```python
from build123d import *

# Parameters (mm, degrees)
BOSS_EXTRUDE1_DEPTH = 16
CUT_EXTRUDE1_START  = 2
CUT_EXTRUDE1_DEPTH  = 14
SKETCH7_R           = 1.625
CUT_EXTRUDE2_DEPTH  = 55.539321396
CUT_EXTRUDE3_START  = -18
SKETCH8_W           = 10.868969255
SKETCH8_H           = 5.55
CUT_EXTRUDE3_DEPTH  = 2.5
SKETCH9_R           = 1.625
CUT_EXTRUDE4_DEPTH  = 8
SKETCH16_R          = 3.75
CUT_EXTRUDE9_DEPTH  = 3
SKETCH21_W          = 35
SKETCH21_H          = 21
CUT_EXTRUDE13_DEPTH = 2
FILLET2_R           = 0.5
FILLET3_R           = 3
FILLET4_R           = 1
CHAMFER3_SIZE       = 3.5
CHAMFER4_SIZE       = 4
SKETCH18_R          = 1.625
CUT_EXTRUDE11_DEPTH = 20
SKETCH19_R          = 4
CUT_EXTRUDE12_DEPTH = 5
CHAMFER9_SIZE       = 2
CHAMFER12_SIZE      = 1.5
CHAMFER11_SIZE      = 2


# Some blends are built 0.0001 mm under size
with BuildPart() as part:
    # Sketch4 → Boss-Extrude1 (new body)
    with BuildSketch(Plane.XY):
        Polygon((-3.5, -0.026126862), (-3.5, 6.973873138), (9, 6.973873138), (9, 12.473873138), (5.5, 12.473873138), (5.5, 27.973873138), (25.5, 27.973873138), (25.5, 15.473873138), (40.5, 15.473873138), (40.5, 9.473873138), (25.5, 9.473873138), (25.5, 6.973873138), (51.5, 6.973873138), (51.5, -0.026126862), align=None)
    extrude(amount=-BOSS_EXTRUDE1_DEPTH)

    # Sketch6 → Cut-Extrude1 (cut)
    with BuildSketch(Plane.XY.offset(CUT_EXTRUDE1_START)):
        with BuildLine():
            Line((12, 19.273873138), (5.5, 19.273873138))
            Line((5.5, 19.273873138), (5.5, 16.973873138))
            Line((5.5, 16.973873138), (20, 16.973873138))
            ThreePointArc((20, 16.973873138), (23.888996032, 18.58469458), (25.499999994, 22.473615007))
            Line((25.499999994, 22.473615007), (25.5, 27.973873138))
            Line((25.5, 27.973873138), (20, 27.973873138))
            ThreePointArc((20, 27.973873138), (17.189181506, 27.201377701), (15.167942816, 25.100891099))
            Line((15.167942816, 25.100891099), (12, 19.273873138))
        make_face()
        with BuildLine():
            Line((20, 18.673873138), (13.608794956, 18.673873138))
            Line((13.608794956, 18.673873138), (16.661487764, 24.28890373))
            ThreePointArc((16.661487764, 24.28890373), (23.26627588, 24.415893189), (20, 18.673873138))
        make_face(mode=Mode.SUBTRACT)
    extrude(amount=-CUT_EXTRUDE1_DEPTH, mode=Mode.SUBTRACT)

    # Sketch7 → Cut-Extrude2 (cut, through all)
    with BuildSketch(Plane(origin=(40.5, 0, 0), x_dir=(0, 0, -1), z_dir=(1, 0, 0))):
        with Locations((8, 12.473873138)):
            Circle(SKETCH7_R)
    extrude(amount=-CUT_EXTRUDE2_DEPTH, mode=Mode.SUBTRACT)

    # Sketch8 → Cut-Extrude3 (cut)
    with BuildSketch(Plane(origin=(40.5, 0, 0), x_dir=(0, 0, -1), z_dir=(1, 0, 0)).offset(CUT_EXTRUDE3_START)):
        with Locations((5.434484628, 12.473873138)):
            Rectangle(SKETCH8_W, SKETCH8_H)
    extrude(amount=-CUT_EXTRUDE3_DEPTH, mode=Mode.SUBTRACT)

    # Sketch9 → Cut-Extrude4 (cut)
    with BuildSketch(Plane.XZ.offset(0.026126862)):
        with Locations((3.5, -8)):
            Circle(SKETCH9_R)
        with Locations((44.5, -8)):
            Circle(SKETCH9_R)
    extrude(amount=-CUT_EXTRUDE4_DEPTH, mode=Mode.SUBTRACT)

    # Sketch16 → Cut-Extrude9 (cut)
    with BuildSketch(Plane(origin=(0, 6.973873138, 0), x_dir=(1, 0, 0), z_dir=(0, 1, 0))):
        with Locations(Location((3.5, 8, 0), (0, 0, 180))):
            Circle(SKETCH16_R)
        with Locations(Location((44.5, 8, 0), (0, 0, 180))):
            Circle(SKETCH16_R)
    extrude(amount=-CUT_EXTRUDE9_DEPTH, mode=Mode.SUBTRACT)

    # Sketch21 → Cut-Extrude13 (cut)
    with BuildSketch(Plane.XY):
        with Locations((23, 17.473873138)):
            Rectangle(SKETCH21_W, SKETCH21_H)
    extrude(amount=-CUT_EXTRUDE13_DEPTH, mode=Mode.SUBTRACT)

    # Fillet2
    fillet2_edges = [part.edges().sort_by_distance(p)[0] for p in [
        (20, 27.973873138, -7),
        (25.499999994, 22.473615007, -7),
    ]]
    fillet(fillet2_edges, radius=FILLET2_R)

    # Fillet3
    fillet3_edges = [part.edges().sort_by_distance(p)[0] for p in [
        (25.5, 27.973873138, -14),
    ]]
    fillet(fillet3_edges, radius=FILLET3_R)

    # Fillet4
    fillet4_edges = [part.edges().sort_by_distance(p)[0] for p in [
        (13.608794956, 18.673873138, -7),
    ]]
    fillet(fillet4_edges, radius=FILLET4_R)

    # Chamfer3
    # the kernel refuses this chamfer: 3.5 mm, written as the material it takes off along each edge
    with BuildSketch(Plane(origin=(5.5, 12.473873138, 7.000890458), x_dir=(-0.02749587661058662, 0.9996219169112968, 0), z_dir=(0, 0, -1))) as chamfer3_piece_1_section:
        Polygon((CHAMFER3_SIZE * 0.999621916911, CHAMFER3_SIZE * 0.0274958766106), (-CHAMFER3_SIZE * 0.0274958766106, CHAMFER3_SIZE * 0.999621916911), (0, 0), align=None)
    chamfer3_piece_1 = extrude(amount=22.376780916, mode=Mode.PRIVATE)
    chamfer3_piece_1 = split(chamfer3_piece_1, bisect_by=Plane(origin=(9, 13.630287679, -4.1875), z_dir=(-1, 0, 0)), keep=Keep.TOP, mode=Mode.PRIVATE)
    add(chamfer3_piece_1, mode=Mode.SUBTRACT)
    with BuildSketch(Plane(origin=(5.5, 12.473873138, -0.624109542), x_dir=(-0.02749587661058662, 0.9996219169112968, 0), z_dir=(0, 0, -1))) as chamfer3_piece_2_section:
        Polygon((CHAMFER3_SIZE * 0.999621916911, CHAMFER3_SIZE * 0.0274958766106), (-CHAMFER3_SIZE * 0.0274958766106, CHAMFER3_SIZE * 0.999621916911), (0, 0), align=None)
    chamfer3_piece_2 = extrude(amount=24.376780916, mode=Mode.PRIVATE)
    chamfer3_piece_2 = split(chamfer3_piece_2, bisect_by=Plane(origin=(9, 13.630287679, -12.8125), z_dir=(-1, 0, 0)), keep=Keep.TOP, mode=Mode.PRIVATE)
    add(chamfer3_piece_2, mode=Mode.SUBTRACT)

    # Chamfer4
    chamfer4_edges = [part.edges().sort_by_distance(p)[0] for p in [
        (5.5, 27.973873138, -9),
    ]]
    chamfer(chamfer4_edges, length=CHAMFER4_SIZE)

    # Sketch18 → Cut-Extrude11 (cut)
    with BuildSketch(Plane.XY):
        with Locations((20, 22.473873138)):
            Circle(SKETCH18_R)
    extrude(amount=-CUT_EXTRUDE11_DEPTH, mode=Mode.SUBTRACT)

    # Sketch19 → Cut-Extrude12 (cut)
    with BuildSketch(Plane(origin=(0, 16.973873138, 0), x_dir=(1, 0, 0), z_dir=(0, 1, 0))):
        with Locations((2.5, 8)):
            Circle(SKETCH19_R)
    extrude(amount=-CUT_EXTRUDE12_DEPTH, mode=Mode.SUBTRACT)

    # Chamfer9
    chamfer9_edges = [part.edges().sort_by_distance(p)[0] for p in [
        (17.25, 6.973873138, -2),
    ]]
    chamfer(chamfer9_edges, length=CHAMFER9_SIZE - 0.0001)  # a hair under: the kernel refuses the full size

    # Chamfer12
    # the kernel refuses this chamfer: 1.5 mm, written as the material it takes off along each edge
    with BuildSketch(Plane(origin=(23.857524482, 18.673873138, -2), x_dir=(0, 0.9996219169112968, 0.027495876610586334), z_dir=(-1, 0, 0))) as chamfer12_piece_1_section:
        Polygon((CHAMFER12_SIZE * 0.999621916911, CHAMFER12_SIZE * 0.0274958766106), (-CHAMFER12_SIZE * 0.0274958766106, CHAMFER12_SIZE * 0.999621916911), (0, 0), align=None)
    chamfer12_piece_1 = extrude(amount=12.424357944, mode=Mode.PRIVATE)
    chamfer12_piece_1 = split(chamfer12_piece_1, bisect_by=Plane(origin=(15.45343037, 22.066839589, -2.289421032), z_dir=(0.8785558517032834, -0.47763962925820797, 0)), keep=Keep.TOP, mode=Mode.PRIVATE)
    add(chamfer12_piece_1, mode=Mode.SUBTRACT)

    # Chamfer11
    chamfer11_edges = [part.edges().sort_by_distance(p)[0] for p in [
        (8.75, 19.273873138, -2),
    ]]
    chamfer(chamfer11_edges, length=CHAMFER11_SIZE)


solid = part.part
```
Here's how the part is built. I have some questions about the finished solid (model axes, mm). A direction names the side the tool comes from. Give positions to 0.01 mm unless a question says otherwise; leave off trailing zeros. Write each loop counter-clockwise with the first axis right and the second up, starting at its lowest first coordinate (ties: lowest second). Pieces come first, ordered by that corner, then holes. Notation, with made-up numbers: M 58,29.25 L 112,29.25 A10 cw 112,35.25 Z; hole C 88,26.5 d1. An arc over 180 degrees is marked long. Put each result on its own line as item: value. Start each with the question number.
Item 1: On a 3-axis mill with a long thin cutter (end or side, diameter ignored), from which of +Z, -Z, +X, -X, +Y, -Y can I reach the whole of each face in a straight line? I mean faces 4 (the flat face through (7.225, 14.248, -8.902)), 5 (the flat face through (21, 15.249, -6)), 6 (the flat face through (11, 25, -2)). Say none if no direction works.
Item 2: If we section it at D-D, the plane x = 4: Write out the boundary of the cut face in (y, z), then the cut area to 3 significant figures.
Item 3: If we section it at B-B, the plane y = 13.25: Write out the boundary of the cut face in (x, z), then the cut area to 3 significant figures.
Item 4: I need wall thicknesses on L1, parallel to Y at x = 36, z = -8; L2, parallel to X at y = 10, z = -10.5; L3, parallel to Y at x = 20, z = -12.25. Which ranges of each line are inside material? Lowest first, please. Write a range as from..to.
Item 5: Will these pins go through, and if not, where does the flat tip stop? pin 1 (3 mm diameter, centred on y = 11.5, z = -8, fed in from +X); pin 2 (3.5 mm diameter, centred on x = 44.5, z = -8, fed in from +Y); pin 3 (3.5 mm diameter, centred on x = 20, y = 22.47, fed in from +Z).
Item 6: Thinking about a two-plate mould opening in X: for faces 1 (the flat face through (51.5, 4, -8)), 2 (the flat face through (18, 18.674, -8)), 3 (the cylindrical face through (15.957, 26.203, -6.93)), which applies, +X half, -X half, draft (parallel to the pull), parting line (faces both ways), or undercut?
Item 7: If we section it at A-A, the plane x = 44.5: Write out the boundary of the cut face in (y, z) (3 decimals).
Item 8: If we section it at C-C, the plane z = -8: Count the separate pieces of the cut face and the enclosed holes in it, then the cut area to 3 significant figures.
Values:
1. face 4: +Z, -Z, -X
1. face 5: +Z
1. face 6: +Z, +X, -X, +Y
2. outline: M -0.03,-16 L 6.97,-16 L 6.97,-11.72 L 3.97,-11.72 L 3.97,-9.55 L -0.03,-9.55 Z; M -0.03,-6.45 L 3.97,-6.45 L 3.97,-4.28 L 6.97,-4.28 L 6.97,0 L -0.03,0 Z
2. area: 77.3 mm²
3. outline: M 8.22,-16 L 40.5,-16 L 40.5,-9.43 L 22.5,-9.43 L 22.5,-10.87 L 20,-10.87 L 20,-9.43 L 8.22,-9.43 Z; M 8.22,-6.57 L 20,-6.57 L 20,-2 L 8.22,-2 Z; M 22.5,-6.57 L 40.5,-6.57 L 40.5,-2 L 22.5,-2 Z
3. area: 345 mm²
4. L1: -0.03..6.97, 9.47..10.85, 14.1..15.47
4. L2: 9..20, 22.5..40.5
4. L3: -0.03..20.85, 24.1..27.97
5. pin 1: x = 40.5
5. pin 2: y = 3.97
5. pin 3: z = -2
6. face 1: +X half
6. face 2: draft
6. face 3: undercut
7. outline: M -0.026,-16 L 6.974,-16 L 6.974,-11.75 L 3.974,-11.75 L 3.974,-9.625 L -0.026,-9.625 Z; M -0.026,-6.375 L 3.974,-6.375 L 3.974,-4.25 L 6.974,-4.25 L 6.974,0 L -0.026,0 Z
8. separate pieces: 6
8. enclosed holes: 1
8. area: 589 mm²
